from build123d import *

# Parameters (mm, degrees)
BOSS_EXTRUDE1_DEPTH                         = 50
BOSS_EXTRUDE2_DEPTH                         = 10
CBORE_FOR_10_BINDING_HEAD_MACHINE_S_2_COUNT = 2
CBORE_FOR_10_BINDING_HEAD_MACHINE_S_2_PITCH = 70.641523205


with BuildPart() as part:
    # Sketch1 → Boss-Extrude1 (new body)
    with BuildSketch(Plane.XY):
        Polygon((0, 110), (10, 110), (10, 10), (60, 10), (60, 0), (0, 0), align=None)
    extrude(amount=BOSS_EXTRUDE1_DEPTH)

    # Sketch2 → Boss-Extrude2 (add)
    with BuildSketch(Plane.XY.offset(50)):
        Polygon((0, 110), (35, 110), (35, 35), (60, 35), (60, 0), (0, 0), align=None)
    extrude(amount=BOSS_EXTRUDE2_DEPTH)

    # Sketch3 → CBORE for #10 Binding Head Machine Screw1 (revolve, cut)
    with BuildSketch(Plane(origin=(17.635166565, 81.246186772, 60), x_dir=(0, -1, 0), z_dir=(1, 0, 0))):
        Polygon((0, 0), (0, 60.000025), (2.5527, 60.000025), (2.5527, 3.1242), (5.55625, 3.1242), (5.55625, 0.635), (6.19125, 0), align=None)
    cbore_for_10_binding_head_machine_screw = revolve(axis=Axis((17.635166565, 81.246186772, 66.35), (0, 0, -1)), mode=Mode.SUBTRACT)

    # CBORE for _10 Binding Head Machine S 2: CBORE for #10 Binding Head Machine Screw1 ×2
    with Locations(*[Vector(0.396309487955917, -0.9181169804312079, 0) * (i * CBORE_FOR_10_BINDING_HEAD_MACHINE_S_2_PITCH) for i in range(1, CBORE_FOR_10_BINDING_HEAD_MACHINE_S_2_COUNT)]):
        add(cbore_for_10_binding_head_machine_screw, mode=Mode.SUBTRACT)


solid = part.part
Read the model definition and answer for the solid it produces. Units are mm, in the model's axes. A direction names the side the tool comes from. Round coordinates to 2 decimals unless told otherwise and drop trailing zeros. Write each loop counter-clockwise with the first axis right and the second up, starting at its lowest first coordinate (ties: lowest second). Pieces come first, ordered by that corner, then holes. Notation, with made-up numbers: (73.25, -35) - (102.25, -35) arc R26 ccw to (102.25, -13) - close; hole circle Ø2 at (54.5, 86). An arc over 180 degrees is marked (long way). Use a Markdown table: item, result.
(1) The part is cut by section A-A (y = 89.5). Write down the section's boundary in (x, z), then the cut area to 3 significant figures.
Reported:
| item | result |
|---|---|
| outline | (0, 0) - (10, 0) - (10, 50) - (35, 50) - (35, 60) - (0, 60) - close |
| area | 850 mm2 |
(2) The mould has two halves that part along Y. Classify faces 5 (the flat face through (47, 35, 55)), 6 (the flat face through (60, 6, 36)), 7 (the cylindrical face through (15.966, 75.947, 58.138)): released by +Y, released by -Y, zero draft, split by the parting line, or undercut.
Reported:
| item | result |
|---|---|
| face 5 | released by +Y |
| face 6 | zero draft |
| face 7 | undercut |
(3) Straight lines are drawn through the part: line 1 along Z through (x, y) = (29, 72.5); line 2 along Y through (x, z) = (34, 9). For each, find the intervals that lie inside material, in ascending order. Write a range as [from, to].
Reported:
| item | result |
|---|---|
| line 1 | [50, 60] |
| line 2 | [0, 10] |
(4) Each of these flat-tipped pins is pushed along its axis until it touches: pin 1 Ø8 at (y, z) = (36, 19.5) entering from +X; pin 2 Ø1.5 at (x, y) = (35.5, 48.5) entering from -Z; pin 3 Ø8 at (y, z) = (58, 55.5) entering from +X. Where does it stop, or does it pass through?
Reported:
| item | result |
|---|---|
| pin 1 | x = 10 |
| pin 2 | z = 50 |
| pin 3 | x = 35 |
(5) Which of the six approach directions +Z, -Z, +X, -X, +Y, -Y give full straight-line access (tool end or side, diameter ignored) to faces 1 (the flat face through (35, 10, 25)), 2 (the flat face through (35, 73, 55)), 3 (the cylindrical face through (43.479, 15.017, 53.486)), 4 (the flat face through (19, 84, 56.876))?
Reported:
| item | result |
|---|---|
| face 1 | -Z, +X, +Y |
| face 2 | +Z, -Z, +X, +Y |
| face 3 | +Z, -Z |
| face 4 | +Z |
